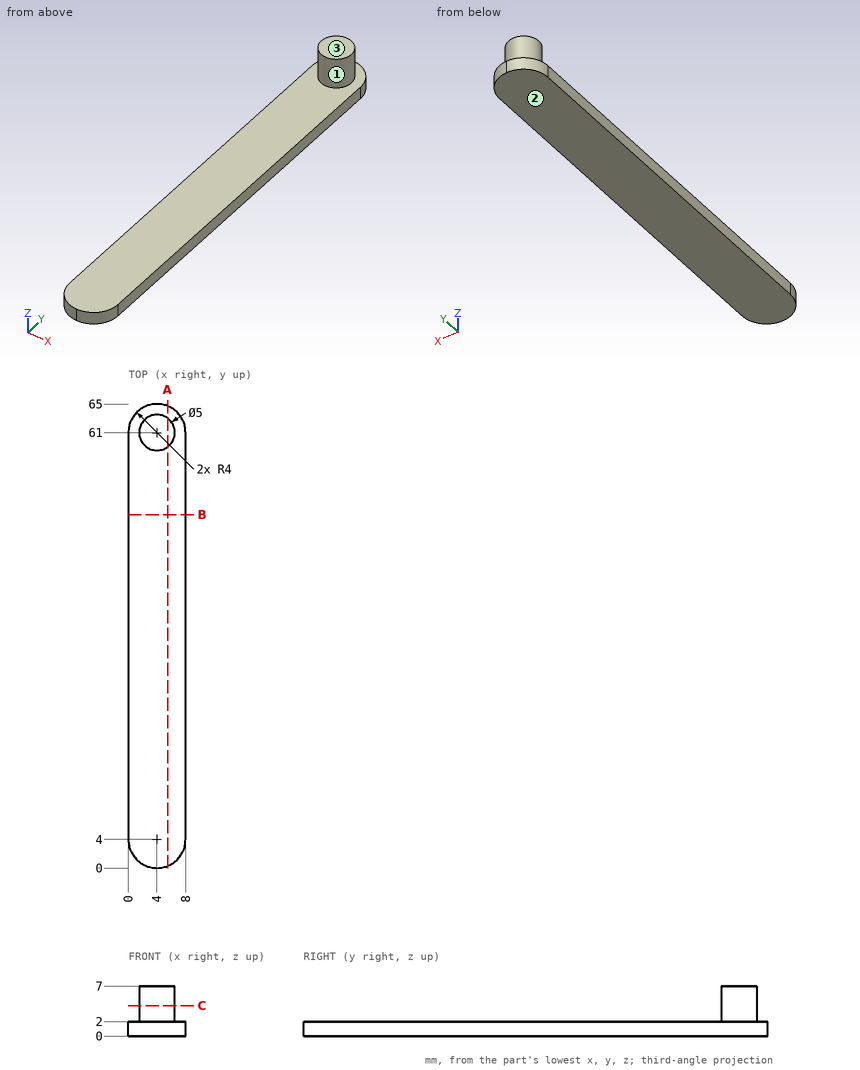
Design review of the part shown in the three views and the two pictorial views. Dimensions are in mm from the part's minimum x, y and z. Round coordinates to 2 decimals unless told otherwise and drop trailing zeros. Write each loop counter-clockwise with the first axis right and the second up, starting at its lowest first coordinate (ties: lowest second). Pieces come first, ordered by that corner, then holes. Notation, with made-up numbers: M -35.5,19 L -8.5,19 A19 ccw -8.5,40 Z; hole C -13,6 d8. An arc over 180 degrees is marked long. One line per item, written item: value. Start each with the question number.
1. Take a section at B-B on y = 49.5. State the section outline as (x, z) points.
2. Clearance check with flat-ended pins moving along their axes: P1, Ø1.5, axis at x = 5, y = 39.5, coming from the +Z side; P2, Ø1.5, axis at x = 3, z = 6, coming from the +Y side. State where each tip first meets the part, or that it passes through.
3. To check wall thickness, follow probe 1 along Z at (x, y) = (5, 47); probe 2 along Y at (x, z) = (4.25, 1.5); probe 3 along Y at (x, z) = (2.5, 5.75). State the ranges of each line that lie inside material, in increasing order. Write a range as from..to.
4. Take a section at C-C on z = 4.25. State the section outline as (x, y) points, then the cut area to 3 significant figures.
5. Draft analysis for pull direction Z (two halves, no side actions). For the marked faces 1, 2 and 3, state which applies: pulls with the +Z half, pulls with the -Z half, needs draft (parallel to the pull), parting line crosses it, or undercut.
6. Take a section at A-A on x = 5.5. State the section outline as (y, z) points, then the cut area to 3 significant figures.
Computed:
1. outline: M 0,0 L 8,0 L 8,2 L 0,2 Z
2. P1: stops at z = 2
2. P2: stops at y = 63.49
3. probe 1: z = 0..2
3. probe 2: y = 0.01..64.99
3. probe 3: y = 59..63
4. outline: C 4,61 d5
4. area: 19.6 mm²
5. face 1: needs draft
5. face 2: pulls with the -Z half
5. face 3: pulls with the +Z half
6. outline: M 0.29,0 L 64.71,0 L 64.71,2 L 63,2 L 63,7 L 59,7 L 59,2 L 0.29,2 Z
6. area: 149 mm²
